Design review of the part shown in the three views and the two pictorial views. Dimensions are in mm from the part's minimum x, y and z. A direction names the side the tool comes from. Give positions to 0.01 mm unless a question says otherwise; leave off trailing zeros. Order: outer loops, then holes, each group sorted by start corner. A loop starts at its lowest first (then second) coordinate and runs counter-clockwise, first axis right, second up.
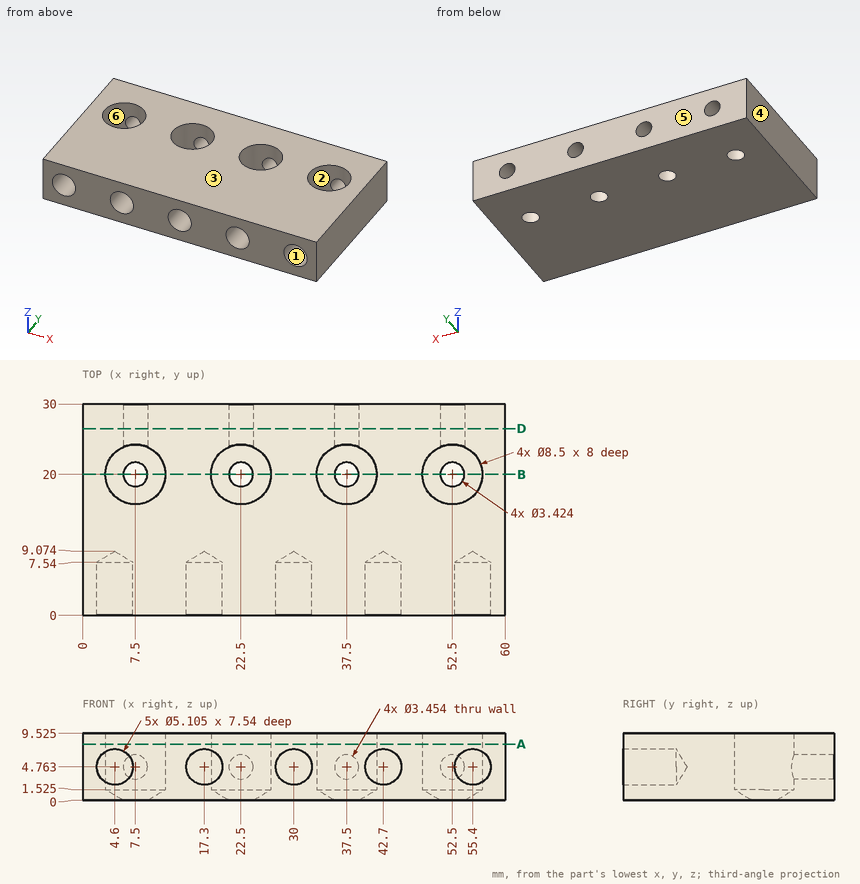
Item 1: Take a section at D-D (y = 26.5). Give the boundary of the cut face in (x, z) (1 decimal), and give its area (3 significant figures).
Values found:
outline: (0, 0) - (60, 0) - (60, 9.5) - (0, 9.5) - close; hole circle Ø3.5 at (7.5, 4.8); hole circle Ø3.5 at (22.5, 4.8); hole circle Ø3.5 at (37.5, 4.8); hole circle Ø3.5 at (52.5, 4.8)
area: 534 mm2
Item 2: For the marked faces 1, 2 and 3, list the 3-axis set-ups (+Z, -Z, +X, -X, +Y, -Y) from which the entire face can be reached by the end or side of a thin tool; tool diameter is ignored.
Values found:
face 1: -Y
face 2: +Z
face 3: +Z, +X, -X, +Y, -Y
Item 3: Take a section at A-A (z = 8). Give the boundary of the cut face in (x, y).
Values found:
outline: (0, 0) - (60, 0) - (60, 30) - (0, 30) - close; hole circle Ø8.5 at (7.5, 20); hole circle Ø8.5 at (22.5, 20); hole circle Ø8.5 at (37.5, 20); hole circle Ø8.5 at (52.5, 20)
Item 4: Take a section at B-B (y = 20). Give the number of separate pieces and of enclosed holes in the cut face, and give its area (3 significant figures).
Values found:
separate pieces: 5
enclosed holes: 0
area: 263 mm2
Item 5: For line 1 (X direction, y = 20, z = 7.5); line 2 (X direction, y = 6, z = 3) (1 decimal); line 3 (X direction, y = 27.5, z = 6.25) (1 decimal), list the stretches that pass through material, from the lowest coordinate up.
Values found:
line 1: x = 0 to 3.25, 11.75 to 18.25, 26.75 to 33.25, 41.75 to 48.25, 56.75 to 60
line 2: x = 0 to 2.8, 6.4 to 15.5, 19.1 to 28.2, 31.8 to 40.9, 44.5 to 53.6, 57.2 to 60
line 3: x = 0 to 6.6, 8.4 to 21.6, 23.4 to 36.6, 38.4 to 51.6, 53.4 to 60
Item 6: Draft analysis for pull direction X (two halves, no side actions). For the marked faces 4, 5 and 6, state which applies: released by +X, released by -X, zero draft, split by the parting line, or undercut.
Values found:
face 4: released by -X
face 5: zero draft
face 6: undercut
Item 7: Clearance check with flat-ended pins moving along their axes: pin 1 Ø3 at (x, z) = (52.5, 4.76) entering from +Y; pin 2 Ø4 at (x, z) = (55.4, 4.76) entering from -Y; pin 3 Ø3 at (x, z) = (17.3, 4.76) entering from -Y. State where each tip first meets the part, or that it passes through.
Values found:
pin 1: stops at y = 16.02
pin 2: stops at y = 7.87
pin 3: stops at y = 8.17
